Verification items for the finished model (mm, model axes). Coordinates: 2 decimals unless noted, no trailing zeros. Loops run counter-clockwise (first coordinate to the right, second up) from the corner with the lowest first, then second, coordinate; pieces in that order, holes last.
Q1. Sectioned sample at A-A (y = 27). Enter the section's corners in (x, z) (3 decimals), then the cut area to 4 significant figures.
Q2. Material ranges on probe 1 along Y at (x, z) = (0, -1.7) (3 decimals); probe 2 along Y at (x, z) = (4.5, -0.25); probe 3 along X at (y, z) = (-6, 0.75), recorded low to high.
Q3. Sectioned sample at B-B (x = -2.5). Count the separate pieces of the cut face and the enclosed holes in it, then the cut area to 3 significant figures.
Q4. Go/stop test with flat-tipped pins: P1, Ø18, axis at x = 0, y = 27, coming from the -Z side; P2, Ø1.5, axis at y = -2.5, z = 0.5, coming from the -X side; P3, Ø4, axis at x = 16, z = -2, coming from the +Y side; P4, Ø4, axis at x = -3.5, z = 0.5, coming from the -Y side. Record where each tip stops, or that it passes through.
```python
from build123d import *

# Parameters (mm, degrees)
F0_R     = 11.125
F1_DEPTH = 3.5
F2_SIZE  = 1
F3_SIZE  = 1


# Not quite as in the source:
# - a feature names something its author has since deleted; it is built from what else it names


with BuildPart() as f1:
    # F0 (on Top) → F1 (new body, symmetric)
    with BuildSketch(Plane.XY):
        with BuildLine():
            ThreePointArc((-1.36e-08, 13.5), (6.7500001307, 11.6913428757), (11.6913431087, 6.7499997269))
            ThreePointArc((11.6913431087, 6.7499997269), (9.8826859022, 13.4999998423), (11.6913429511, 20.25))
            ThreePointArc((11.6913429511, 20.25), (6.7499999941, 15.3086570455), (-1.36e-08, 13.5))
        make_face()
        with BuildLine():
            ThreePointArc((-11.691342964, 6.7499999776), (-6.7500000171, 11.6913429412), (-1.36e-08, 13.5))
            ThreePointArc((-1.36e-08, 13.5), (-6.7500000059, 15.3086570523), (-11.6913429511, 20.25))
            ThreePointArc((-11.6913429511, 20.25), (-9.8826859022, 13.4999999871), (-11.691342964, 6.7499999776))
        make_face()
        with BuildLine():
            ThreePointArc((-11.6913429875, -6.749999937), (-13.5, 2.34e-08), (-11.691342964, 6.7499999776))
            ThreePointArc((-11.691342964, 6.7499999776), (-16.6326859134, 1.8086570424), (-23.3826859022, 0))
            ThreePointArc((-23.3826859022, 0), (-16.6326859337, -1.8086570307), (-11.6913429875, -6.749999937))
        make_face()
        with BuildLine():
            ThreePointArc((-11.6913429511, -20.25), (-6.7500000035, -15.3086570509), (-8.1e-09, -13.5))
            ThreePointArc((-8.1e-09, -13.5), (-6.750000035, -11.6913429309), (-11.6913429875, -6.749999937))
            ThreePointArc((-11.6913429875, -6.749999937), (-10.3426872567, -10.005942856), (-9.8826859022, -13.5))
            ThreePointArc((-9.8826859022, -13.5), (-10.3426872473, -16.9940571089), (-11.6913429511, -20.25))
        make_face()
        with BuildLine():
            ThreePointArc((11.6913429511, -20.25), (9.8826859022, -13.5000001869), (11.6913427641, -6.7500003238))
            ThreePointArc((11.6913427641, -6.7500003238), (6.7499998346, -11.6913430466), (-8.1e-09, -13.5))
            ThreePointArc((-8.1e-09, -13.5), (6.7499999965, -15.3086570469), (11.6913429511, -20.25))
        make_face()
        with BuildLine():
            ThreePointArc((11.6913431087, 6.7499997269), (13.0399986957, 3.4940569566), (13.5, 0))
            ThreePointArc((13.5, 0), (13.0399986065, -3.4940572895), (11.6913427641, -6.7500003238))
            ThreePointArc((11.6913427641, -6.7500003238), (16.6326857403, -1.8086571424), (23.3826859022, 0))
            ThreePointArc((23.3826859022, 0), (16.6326860387, 1.8086569701), (11.6913431087, 6.7499997269))
        make_face()
        with BuildLine():
            ThreePointArc((11.6913427641, -6.7500003238), (13.0399986065, -3.4940572895), (13.5, 0))
            ThreePointArc((13.5, 0), (13.0399986957, 3.4940569566), (11.6913431087, 6.7499997269))
            ThreePointArc((11.6913431087, 6.7499997269), (6.7500001307, 11.6913428757), (-1.36e-08, 13.5))
            ThreePointArc((-1.36e-08, 13.5), (-6.7500000171, 11.6913429412), (-11.691342964, 6.7499999776))
            ThreePointArc((-11.691342964, 6.7499999776), (-13.5, 2.34e-08), (-11.6913429875, -6.749999937))
            ThreePointArc((-11.6913429875, -6.749999937), (-6.750000035, -11.6913429309), (-8.1e-09, -13.5))
            ThreePointArc((-8.1e-09, -13.5), (6.7499998346, -11.6913430466), (11.6913427641, -6.7500003238))
        make_face()
        Circle(F0_R, mode=Mode.SUBTRACT)
        with BuildLine():
            ThreePointArc((-11.6913429511, 20.25), (-6.7500000059, 15.3086570523), (-1.36e-08, 13.5))
            ThreePointArc((-1.36e-08, 13.5), (6.7499999941, 15.3086570455), (11.6913429511, 20.25))
            ThreePointArc((11.6913429511, 20.25), (13.0399986549, 23.5059428911), (13.5, 27))
            ThreePointArc((13.5, 27), (-3.4940571089, 40.0399986549), (-11.6913429511, 20.25))
        make_face()
        with Locations((0, 27)):
            Circle(F0_R, mode=Mode.SUBTRACT)
        with BuildLine():
            ThreePointArc((-9.8826859022, -13.5), (-10.3426872567, -10.005942856), (-11.6913429875, -6.749999937))
            ThreePointArc((-11.6913429875, -6.749999937), (-16.6326859337, -1.8086570307), (-23.3826859022, 0))
            ThreePointArc((-23.3826859022, 0), (-35.0740288533, -20.25), (-11.6913429511, -20.25))
            ThreePointArc((-11.6913429511, -20.25), (-10.3426872473, -16.9940571089), (-9.8826859022, -13.5))
        make_face()
        with Locations((-23.3826859022, -13.5)):
            Circle(F0_R, mode=Mode.SUBTRACT)
        with BuildLine():
            ThreePointArc((23.3826859022, 0), (16.6326857403, -1.8086571424), (11.6913427641, -6.7500003238))
            ThreePointArc((11.6913427641, -6.7500003238), (9.8826859022, -13.5000001869), (11.6913429511, -20.25))
            ThreePointArc((11.6913429511, -20.25), (26.8767430111, -26.5399986549), (36.8826859022, -13.5))
            ThreePointArc((36.8826859022, -13.5), (32.9286274482, -3.954058454), (23.3826859022, 0))
        make_face()
        with Locations((23.3826859022, -13.5)):
            Circle(F0_R, mode=Mode.SUBTRACT)
    extrude(amount=F1_DEPTH, both=True)

    # F2
    f2_edges = [f1.edges().sort_by_distance(p)[0] for p in [
        (-11.125, 0, 3.5),
        (-11.125, 27, 3.5),
        (-34.507686, -13.5, 3.5),
        (12.257686, -13.5, 3.5),
    ]]
    chamfer(f2_edges, length=F2_SIZE)

    # F3
    f3_edges = [f1.edges().sort_by_distance(p)[0] for p in [
        (-11.125, 0, -3.5),
        (-11.125, 27, -3.5),
        (-34.507686, -13.5, -3.5),
        (12.257686, -13.5, -3.5),
    ]]
    chamfer(f3_edges, length=F3_SIZE)


solid = f1.part
```
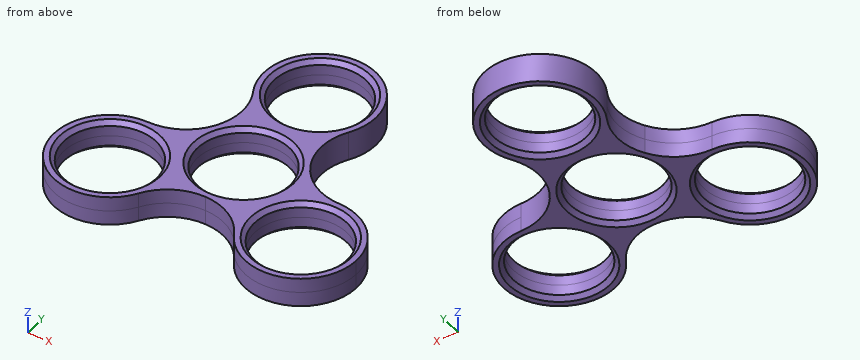
Geometry check:
1. outline: (-13.5, -3.5) - (-12.125, -3.5) - (-11.125, -2.5) - (-11.125, 2.5) - (-12.125, 3.5) - (-13.5, 3.5) - close; (11.125, -2.5) - (12.125, -3.5) - (13.5, -3.5) - (13.5, 3.5) - (12.125, 3.5) - (11.125, 2.5) - close
1. area: 31.25 mm2
2. probe 1: y = -13.5 to -11.125, 11.125 to 15.875, 38.125 to 40.5
2. probe 2: y = -14.27 to -10.17, 10.17 to 16.83, 37.17 to 39.73
2. probe 3: x = -34.61 to -31.6, -15.17 to -9.37, 9.37 to 15.17, 31.6 to 34.61
3. separate pieces: 3
3. enclosed holes: 0
3. area: 70.4 mm2
4. P1: passes through
4. P2: stops at x = -32.17
4. P3: stops at y = 3.79
4. P4: stops at y = -14.67
